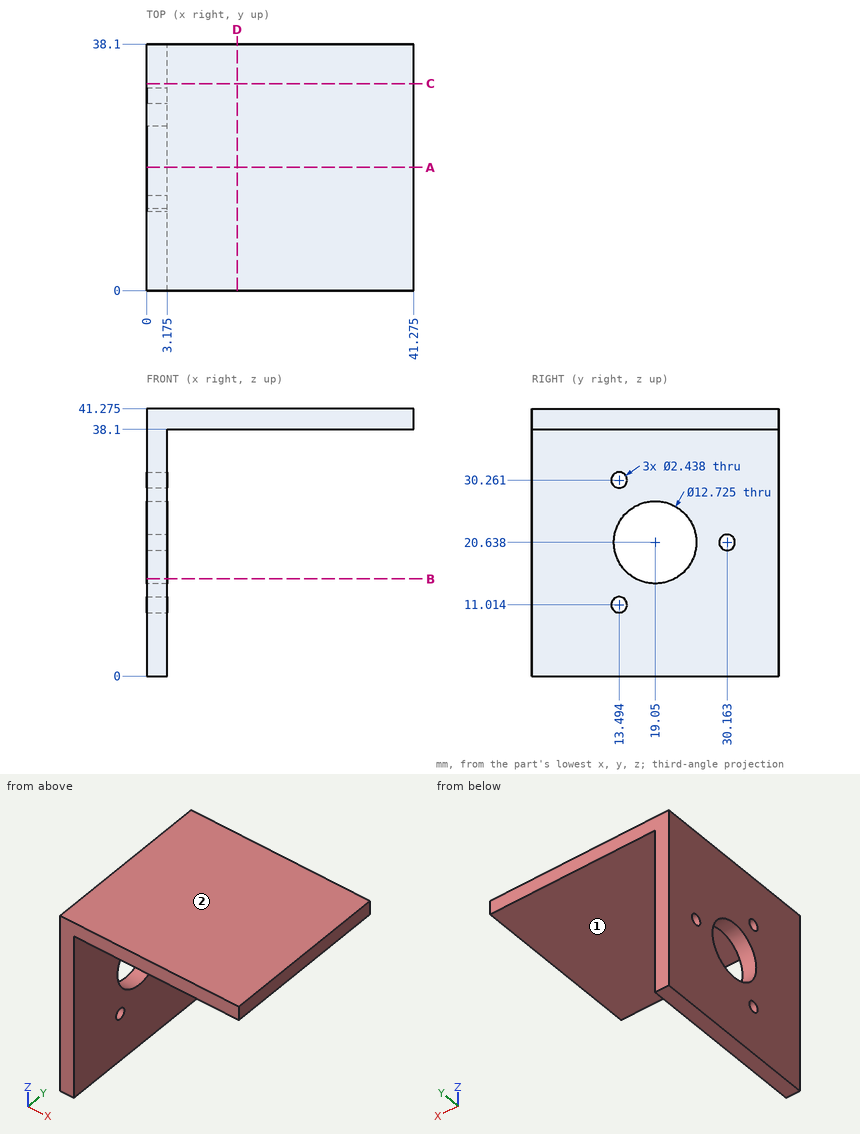
Print and shaded views of the part. All mm, measured from the part's lowest x, y and z. A direction names the side the tool comes from. Coordinates: 2 decimals unless noted, no trailing zeros. Write each loop counter-clockwise with the first axis right and the second up, starting at its lowest first coordinate (ties: lowest second). Pieces come first, ordered by that corner, then holes.
(1) 3-axis set-ups, long thin cutter, end or side, ignore diameter. For the marked faces 1 and 2: which of +Z, -Z, +X, -X, +Y, -Y reach the whole face in a straight line?
(2) Cut at B-B, the plane z = 15. List the corners of the cut face in (x, y) (1 decimal), and give its area (3 significant figures).
(3) Cut at C-C, the plane y = 32. List the corners of the cut face in (x, z) (1 decimal), and give its area (3 significant figures).
(4) Cut at D-D, the plane x = 14. List the corners of the cut face in (y, z) (1 decimal).
(5) Cut at A-A, the plane y = 19.05. List the corners of the cut face in (x, z) (1 decimal).
(6) Drill centre lines: probe 1 along Z at (x, y) = (16, 8) (1 decimal); probe 2 along X at (y, z) = (34, 9.5) (1 decimal). Where is each one in solid material? Low to high.
(7) Flat gauge pins, fed straight in: pin 1 (16.5 mm diameter, centred on y = 19.05, z = 20.64, fed in from +X) (1 decimal); pin 2 (6 mm diameter, centred on x = 20, y = 21, fed in from -Z). Where does each tip first touch, or does it go through?
Geometry says:
1. face 1: -Z, +X, +Y, -Y
1. face 2: +Z, +X, -X, +Y, -Y
2. outline: (0, 0) - (3.2, 0) - (3.2, 16.1) - (0, 16.1) - close; (0, 22) - (3.2, 22) - (3.2, 38.1) - (0, 38.1) - close
2. area: 102 mm2
3. outline: (0, 0) - (3.2, 0) - (3.2, 38.1) - (41.3, 38.1) - (41.3, 41.3) - (0, 41.3) - close
3. area: 252 mm2
4. outline: (0, 38.1) - (38.1, 38.1) - (38.1, 41.3) - (0, 41.3) - close
5. outline: (0, 0) - (3.2, 0) - (3.2, 14.3) - (0, 14.3) - close; (0, 27) - (3.2, 27) - (3.2, 38.1) - (41.3, 38.1) - (41.3, 41.3) - (0, 41.3) - close
6. probe 1: z = 38.1 to 41.3
6. probe 2: x = 0 to 3.2
7. pin 1: stops at x = 3.2
7. pin 2: stops at z = 38.1
